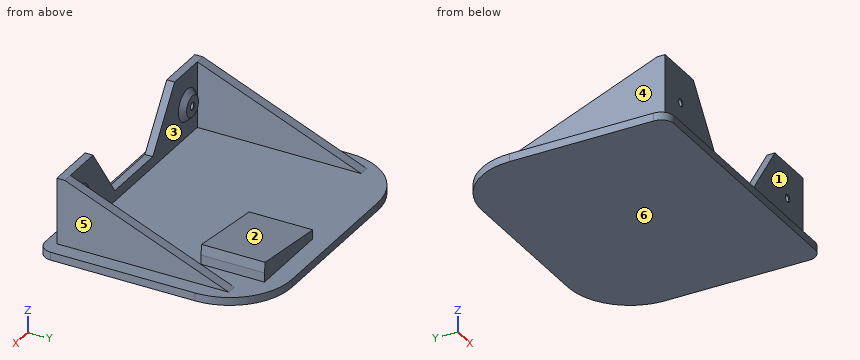
```python
from build123d import *

# Parameters (mm, degrees)
PLATE_DEPTH               = 3
BRACKET_DEPTH             = 46.5
BRACKET_HOLLOW_DEPTH      = 42.75
SKETCH29_R                = 4
INSERT_BOSS_DEPTH         = 2
INSERT_CHAMFER_SIZE       = 2
M3_MOUNT_HOLES_AT_2_COUNT = 2
M3_MOUNT_HOLES_AT_2_PITCH = 72
CUT_EXTRUDE1_DEPTH        = 97.489126654
TOP_CAM_BOSS_START        = 15
TOP_CAM_BOSS_DEPTH        = 24


with BuildPart() as part:
    # Sketch1 → plate (new body)
    with BuildSketch(Plane.XY):
        with BuildLine():
            Line((-28.8875, 46.0375), (28.8875, 46.0375))
            ThreePointArc((28.8875, 46.0375), (45.504509358, 39.154509358), (52.3875, 22.5375))
            Line((52.3875, 22.5375), (52.3875, 0))
            Line((52.3875, 0), (52.3875, -32))
            ThreePointArc((52.3875, -32), (50.923033906, -35.535533906), (47.3875, -37))
            Line((47.3875, -37), (-47.3875, -37))
            ThreePointArc((-47.3875, -37), (-50.923033906, -35.535533906), (-52.3875, -32))
            Line((-52.3875, -32), (-52.3875, 0))
            Line((-52.3875, 0), (-52.3875, 22.5375))
            ThreePointArc((-52.3875, 22.5375), (-45.504509358, 39.154509358), (-28.8875, 46.0375))
        make_face()
    extrude(amount=PLATE_DEPTH)

    # Sketch9 → bracket (add, symmetric)
    with BuildSketch(Plane(origin=(0, 0, 0), x_dir=(0, 0, -1), z_dir=(1, 0, 0))):
        Polygon((-3, 32), (-3, -33), (-28, -33), (-28, -30), align=None)
    extrude(amount=BRACKET_DEPTH, both=True)

    # Sketch10 → bracket hollow (cut, symmetric)
    with BuildSketch(Plane(origin=(0, 0, 0), x_dir=(0, 0, -1), z_dir=(1, 0, 0))):
        Polygon((-28, -30), (-3, -30), (-3, 32), align=None)
    extrude(amount=BRACKET_HOLLOW_DEPTH, both=True, mode=Mode.SUBTRACT)

    # Sketch29 → insert boss (add)
    with BuildSketch(Plane(origin=(0, -30, 0), x_dir=(1, 0, 0), z_dir=(0, 1, 0))):
        with Locations(Location((36, -15, 0), (0, 0, 90))):
            Circle(SKETCH29_R)
        with Locations(Location((-36, -15, 0), (0, 0, 90))):
            Circle(SKETCH29_R)
    extrude(amount=INSERT_BOSS_DEPTH)

    # insert chamfer
    insert_chamfer_edges = [part.edges().sort_by_distance(p)[0] for p in [
        (36, -30, 19),
        (-36, -30, 19),
    ]]
    chamfer(insert_chamfer_edges, length=INSERT_CHAMFER_SIZE - 0.0001)  # a hair under: the kernel refuses the full size

    # Sketch12 → M3 mount holes (revolve, cut)
    with BuildSketch(Plane(origin=(36, -33, 15), x_dir=(0, 0, -1), z_dir=(1, 0, 0))):
        Polygon((0, 0), (0, 5), (1.5, 5), (1.25, 4.75), (1.25, 0.25), (1.5, 0), align=None)
    m3_mount_holes = revolve(axis=Axis((36, -39.35, 15), (0, 1, 0)), mode=Mode.SUBTRACT)

    # M3 mount holes at 2: M3 mount holes ×2
    with Locations(*[(-i * M3_MOUNT_HOLES_AT_2_PITCH, 0, 0) for i in range(1, M3_MOUNT_HOLES_AT_2_COUNT)]):
        add(m3_mount_holes, mode=Mode.SUBTRACT)

    # Sketch30 → Cut-Extrude1 (cut, through all)
    with BuildSketch(Plane(origin=(0, -30, 0), x_dir=(1, 0, 0), z_dir=(0, 1, 0))):
        Polygon((-27.5, -28), (-12.795641698, -7), (12.795641698, -7), (27.5, -28), align=None)
    extrude(amount=-CUT_EXTRUDE1_DEPTH, mode=Mode.SUBTRACT)

    # Sketch5 → top-cam-boss (add)
    with BuildSketch(Plane(origin=(0, 0, 0), x_dir=(1, 0, 0), z_dir=(0, 1, 0)).offset(TOP_CAM_BOSS_START)):
        Polygon((2.5, -6.5), (34.5, -10.315768982), (34.955002904, -6.5), (34.955002904, -3), (2.5, -3), align=None)
    extrude(amount=TOP_CAM_BOSS_DEPTH)


solid = part.part
```
Can you work these out from the model? Positions are in its coordinate system, mm. Face numbers are marked on the shaded views. A direction names the side the tool comes from. Give positions to 0.01 mm unless a question says otherwise; leave off trailing zeros. Loops run counter-clockwise (first coordinate to the right, second up) from the corner with the lowest first, then second, coordinate; pieces in that order, holes last. Notation, with made-up numbers: M 25.25,0.5 L 76.25,0.5 A30 ccw 76.25,27.5 Z; hole C 6,76.5 d2. An arc over 180 degrees is marked long. Use one line per item in the form item = value. Start each with the question number.
(1) On a 3-axis mill with a long thin cutter (end or side, diameter ignored), from which of +Z, -Z, +X, -X, +Y, -Y can I reach the whole of each face in a straight line? I mean the marked faces 1 and 2. Say none if no direction works.
(2) I want a section at D-D, the plane x = 4. Write out the boundary of the cut face in (y, z), and give its area (3 significant figures).
(3) Thinking about a two-plate mould opening in X: for the marked faces 3, 4, 5 and 6, which applies, released by +X, released by -X, zero draft, split by the parting line, or undercut?
(4) Please list where these lines run through material, in increasing order: line 1 (Y direction, x = 29.5, z = 7); line 2 (X direction, y = 1, z = 4.5); line 3 (X direction, y = -31.75, z = 15).
(5) I want a section at A-A, the plane z = 23.5. Write out the boundary of the cut face in (x, y), and give its area (3 significant figures).
(6) I'm going to push flat-ended pins straight in: P1, Ø7.5, axis at y = -3.5, z = 20.5, coming from the -X side; P2, Ø2, axis at x = 16.5, z = 5, coming from the -Y side; P3, Ø1, axis at y = -25.5, z = 22.5, coming from the +X side. Where does each tip first touch, or does it pass through?
(7) I want a section at C-C, the plane y = -21. Write out the boundary of the cut face in (x, z), and give its area (3 significant figures).
Worked out:
q1.face_1 = +Z, +X, -X, -Y
q1.face_2 = +Z, +Y
q2.outline = M -37,0 L 46.04,0 L 46.04,3 L 39,3 L 39,6.68 L 15,6.68 L 15,3 L -30,3 L -30,7 L -33,7 L -33,3 L -37,3 Z
q2.area = 349 mm²
q3.face_3 = undercut
q3.face_4 = released by -X
q3.face_5 = released by +X
q3.face_6 = zero draft
q4.line_1 = -33 to -30, 15 to 39
q4.line_2 = -46.5 to -42.75, 42.75 to 46.5
q4.line_3 = -46.5 to -37.25, -34.75 to -18.4, 18.4 to 34.75, 37.25 to 46.5
q5.outline = M -46.5,-33 L -24.35,-33 L -24.35,-30 L -42.75,-30 L -42.75,-18.84 L -46.5,-18.84 Z; M 24.35,-33 L 46.5,-33 L 46.5,-18.84 L 42.75,-18.84 L 42.75,-30 L 24.35,-30 Z
q5.area = 217 mm²
q6.P1 = -46.5
q6.P2 = -33
q6.P3 = 46.5
q7.outline = M -52.39,0 L 52.39,0 L 52.39,3 L 46.5,3 L 46.5,24.37 L 42.75,24.37 L 42.75,3 L -42.75,3 L -42.75,24.37 L -46.5,24.37 L -46.5,3 L -52.39,3 Z
q7.area = 475 mm²
